Part model, mm, in its own coordinate system. Face numbers are marked on the shaded views. A direction names the side the tool comes from. Give positions to 0.01 mm unless a question says otherwise; leave off trailing zeros. Write each loop counter-clockwise with the first axis right and the second up, starting at its lowest first coordinate (ties: lowest second). Pieces come first, ordered by that corner, then holes. Notation, with made-up numbers: M 29,34.25 L 48,34.25 A18 cw 48,55.25 Z; hole C -38.75,24 d10. An arc over 180 degrees is marked long. Answer as CSV lines item,"result". Start each with the question number.
Item 1: Band-saw the part on A-A, the plane x = 0. List the corners of the cut face in (y, z), then the cut area to 3 significant figures.
Item 2: Pin check, flat tips, straight feed: pin 1 (7 mm diameter, centred on x = 0, y = 0, fed in from -Z); pin 2 (1.8 mm diameter, centred on x = -1.5, y = 0.5, fed in from -Z); pin 3 (1 mm diameter, centred on y = 5, z = 9, fed in from -X) (3 decimals). Stop position of each tip, or through.
Item 3: 3-axis set-ups, long thin cutter, end or side, ignore diameter. For the marked faces 4 and 5: which of +Z, -Z, +X, -X, +Y, -Y reach the whole face in a straight line?
Item 4: Wall check: L1, parallel to Y at x = 0, z = 0.9; L2, parallel to Y at x = 0, z = 7; L3, parallel to Z at x = 3.5, y = 2. Give the ranges that are in metal, low to high. Write a range as from..to.
Item 5: Band-saw the part on B-B, the plane z = 3.5. List the corners of the cut face in (x, y).
Item 6: Two-plate mould, pull along Y, no slides. Class the marked faces 1, 2 and 3: +Y half, -Y half, draft (parallel to the pull), parting line (faces both ways), or undercut.
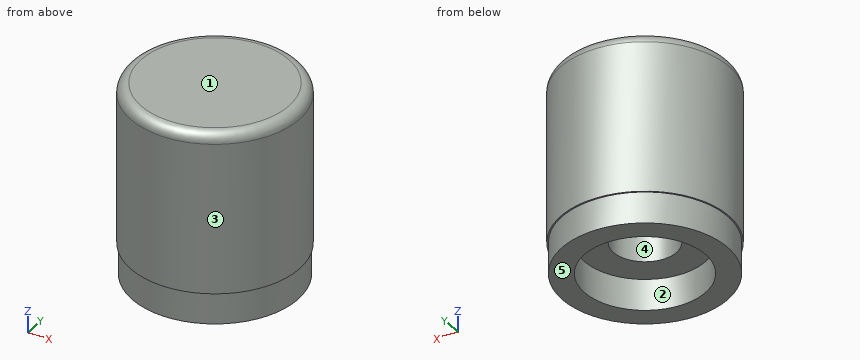
Autodesk Inventor part; units mm, degrees
ref_plane "YZ Plane" through (0, 0, 0) normal (1, 0, 0) x (0, 1, 0)
ref_plane "XZ Plane" through (0, 0, 0) normal (0, 1, 0) x (-1, 0, 0)
ref_plane "XY Plane" through (0, 0, 0) normal (0, 0, 1) x (1, 0, 0)
sketch "Skizze1" plane through (0, 0, 0) normal (0, 0, 1) x (1, 0, 0)
  circle A0 centre (0, 0) radius 8.5
  circle A1 centre (0, 0) radius 3.7
  circle A2 centre (0, 0) radius 8
  circle A3 centre (0, 0) radius 5.85
  point P0 (0, 0)
  dimension "d0" = 16
  dimension "d1" = 11.7
extrude "Extrusion1" add sketch "Skizze1" along normal blind 3 contours A2
sketch "Skizze2" plane through (0, 0, 3) normal (0, 0, 1) x (1, 0, 0)
  circle A0 centre (0, 0) radius 3.05
  circle A1 centre (0, 0) radius 8.1333
  dimension "d4" = 6.1
extrude "Extrusion2" add sketch "Skizze2" along normal blind 15
sketch "Skizze3" plane through (0, 0, 18) normal (0, 0, 1) x (1, 0, 0)
  circle A0 centre (0, 0) radius 8.1333
extrude "Extrusion3" add sketch "Skizze3" along normal blind 0.5
fillet "Rundung1" radius 1 1 edges at (-8.1333, 0, 18.5)
properties part number "Knopp"
Output:
1,outline,"M -8.13,3 L -8,3 L -8,0 L -5.85,0 L -5.85,3 L -3.05,3 L -3.05,18 L 3.05,18 L 3.05,3 L 5.85,3 L 5.85,0 L 8,0 L 8,3 L 8.13,3 L 8.13,17.5 A1 ccw 7.13,18.5 L -7.13,18.5 A1 ccw -8.13,17.5 Z"
1,area,"173 mm²"
2,pin 1,"z = 3"
2,pin 2,"z = 18"
2,pin 3,"x = -6.775"
3,face 4,"-Z"
3,face 5,"-Z, +X, -X, +Y, -Y"
4,L1,"-8..-5.85, 5.85..8"
4,L2,"-8.13..-3.05, 3.05..8.13"
4,L3,"3..18.5"
5,outline,"C 0,0 d16.27; hole C 0,0 d6.1"
6,face 1,"draft"
6,face 2,"undercut"
6,face 3,"parting line"
